Build history of the part. All positions in model axes, mm. A direction names the side the tool comes from. Give positions to 0.01 mm unless a question says otherwise; leave off trailing zeros. Order: outer loops, then holes, each group sorted by start corner. A loop starts at its lowest first (then second) coordinate and runs counter-clockwise, first axis right, second up. Notation, with made-up numbers: (64.5, -39.5) - (107.5, -39.5) arc R16 ccw to (107.5, -22.5) - close; hole circle Ø5 at (40.25, 48). An arc over 180 degrees is marked (long way). Use a Markdown table: item, result. Add a question column.
(1) Slice it at A-A (z = 10.25). Write the cut outline in (x, y) (1 decimal), then the cut area to 3 significant figures.
(2) Slice it at B-B (y = 9). Write the cut outline in (x, z).
(3) Slice it at D-D (y = 32). Write the cut outline in (x, z), then the cut area to 3 significant figures.
(4) Slice it at C-C (x = 79). Write the cut outline in (y, z) (3 decimals).
(5) Wall check: line 1 (Z direction, x = 48, y = 51); line 2 (X direction, y = 50.5, z = 5.25); line 3 (X direction, y = 26.5, z = 13.25). Give the ranges that are in metal, low to high.
(6) Mould opens along X. For faces 1 (the face through (152.53, 14.13, 21.73)), 2 (the face through (16, 28, 22.22)), 3 (the face through (177.69, 41.12, 21.71)), 4 (the face through (3.541, 41.627, 10.461)) say: +X half, -X half, draft (parallel to the pull), parting line (faces both ways), or undercut.
(7) Which spindle directions (+Z, -Z, +X, -X, +Y, -Y) get a long thin tool onto all of the face, cutting with end or side? Do faces 5 (the face through (28.987, 13.742, 21.727)), 6 (the face through (177.577, 13.742, 21.727)), 7 (the face through (29.576, 41.24, 12.069)). Say none if no direction does.
(8) Flat gauge pins, fed straight in: pin 1 (1.5 mm diameter, centred on y = 17, z = 16, fed in from -X); pin 2 (1.5 mm diameter, centred on y = 44.5, z = 6.5, fed in from +X); pin 3 (12 mm diameter, centred on y = 14, z = 20, fed in from -X). Where does each tip first touch, or does it go through?
from build123d import *

# Parameters (mm, degrees)
EXTRUDE001_DEPTH = 19.05
EXTRUDE_DEPTH    = 3.17
CHAMFER_SIZE     = 1


with BuildPart() as extrude001:
    # Sketch001 (on Face8 of Extrude) → Extrude001 (new body)
    with BuildSketch(Plane.XY.offset(3.17)):
        Polygon((6.985, 55.245), (0, 27.6225), (6.985, 0), (26.035, 0), (33.02, 27.6225), (26.035, 55.245), align=None)
        Polygon((174.625, 55.245), (155.575, 55.245), (148.59, 27.6225), (155.575, 0), (174.625, 0), (181.61, 27.6225), align=None)
    extrude(amount=EXTRUDE001_DEPTH)


with BuildPart() as chamfer_body:
    # Sketch → Extrude (new body)
    with BuildSketch(Plane.XY):
        Polygon((6.985, 0), (174.625, 0), (181.61, 27.6225), (174.625, 55.245), (6.985, 55.245), (0, 27.6225), align=None)
    extrude(amount=EXTRUDE_DEPTH)

    # Fusion: union Extrude001
    add(extrude001.part)

    # Chamfer
    chamfer_edges = [chamfer_body.edges().sort_by_distance(p)[0] for p in [
        (16.51, 0, 22.22),
        (165.1, 0, 22.22),
        (3.4925, 13.81125, 22.22),
        (178.1175, 13.81125, 22.22),
        (29.5275, 13.81125, 22.22),
        (3.4925, 41.43375, 22.22),
        (29.5275, 41.43375, 22.22),
        (16.51, 55.245, 22.22),
        (152.0825, 41.43375, 22.22),
        (152.0825, 13.81125, 22.22),
        (165.1, 55.245, 22.22),
        (178.1175, 41.43375, 22.22),
    ]]
    chamfer(chamfer_edges, length=CHAMFER_SIZE)


solid = chamfer_body.part
Solution:
| question | item | result |
|---|---|---|
| 1 | outline | (0, 27.6) - (7, 0) - (26, 0) - (33, 27.6) - (26, 55.2) - (7, 55.2) - close; (148.6, 27.6) - (155.6, 0) - (174.6, 0) - (181.6, 27.6) - (174.6, 55.2) - (155.6, 55.2) - close |
| 1 | area | 2,880 mm2 |
| 2 | outline | (4.71, 0) - (176.9, 0) - (176.9, 21.22) - (175.87, 22.22) - (154.33, 22.22) - (153.3, 21.22) - (153.3, 3.17) - (28.31, 3.17) - (28.31, 21.22) - (27.28, 22.22) - (5.74, 22.22) - (4.71, 21.22) - close |
| 3 | outline | (1.11, 0) - (180.5, 0) - (180.5, 21.22) - (179.47, 22.22) - (150.73, 22.22) - (149.7, 21.22) - (149.7, 3.17) - (31.91, 3.17) - (31.91, 21.22) - (30.88, 22.22) - (2.14, 22.22) - (1.11, 21.22) - close |
| 3 | area | 1,740 mm2 |
| 4 | outline | (0, 0) - (55.245, 0) - (55.245, 3.17) - (0, 3.17) - close |
| 5 | line 1 | 0 to 3.17 |
| 5 | line 2 | 5.79 to 27.23, 154.38 to 175.82 |
| 5 | line 3 | 0.28 to 32.74, 148.87 to 181.33 |
| 6 | face 1 | undercut |
| 6 | face 2 | draft |
| 6 | face 3 | +X half |
| 6 | face 4 | -X half |
| 7 | face 5 | +Z, -Y |
| 7 | face 6 | +Z, +X, -Y |
| 7 | face 7 | +Z, +Y |
| 8 | pin 1 | x = 2.5 |
| 8 | pin 2 | x = 177.53 |
| 8 | pin 3 | x = 1.93 |
